from build123d import *

# Parameters (mm, degrees)
SKETCH1_W               = 100
SKETCH1_H               = 150
SKETCH1_W_2             = 88
SKETCH1_H_2             = 138
BOSS_EXTRUDE1_DEPTH     = 138.202315188
SKETCH2_R               = 40
CUT_EXTRUDE1_DEPTH      = 51
CUT_EXTRUDE1_DEPTH_BACK = 51


with BuildPart() as part:
    # Sketch1 → Boss-Extrude1 (new body)
    with BuildSketch(Plane.XY):
        Rectangle(SKETCH1_W, SKETCH1_H)
        Rectangle(SKETCH1_W_2, SKETCH1_H_2, mode=Mode.SUBTRACT)
    extrude(amount=BOSS_EXTRUDE1_DEPTH)

    # Sketch2 → Cut-Extrude1 (cut, two sides)
    with BuildSketch(Plane(origin=(0, 0, 0), x_dir=(0, 0, -1), z_dir=(1, 0, 0))) as cut_extrude1_sk:
        Circle(SKETCH2_R)
    extrude(amount=CUT_EXTRUDE1_DEPTH, mode=Mode.SUBTRACT)
    extrude(cut_extrude1_sk.sketch, amount=-CUT_EXTRUDE1_DEPTH_BACK, mode=Mode.SUBTRACT)


solid = part.part
Verification items for the finished model (mm, model axes). A direction names the side the tool comes from. Give positions to 0.01 mm unless a question says otherwise; leave off trailing zeros. Loops run counter-clockwise (first coordinate to the right, second up) from the corner with the lowest first, then second, coordinate; pieces in that order, holes last. Notation, with made-up numbers: (75.25, 50.25) - (104.25, 50.25) arc R31 cw to (104.25, 81.25) - close; hole circle Ø3 at (67.25, 45.25). An arc over 180 degrees is marked (long way). Write each question's results on one line, items separated by ' | '.
1) Sectioned sample at A-A on z = 24. Record the boundary of the cut face in (x, y), plus the area to 3 significant figures.
Solution:
outline: (-50, -75) - (50, -75) - (50, -32) - (44, -32) - (44, -69) - (-44, -69) - (-44, -32) - (-50, -32) - close; (-50, 32) - (-44, 32) - (-44, 69) - (44, 69) - (44, 32) - (50, 32) - (50, 75) - (-50, 75) - close | area: 2,090 mm2
2) Sectioned sample at B-B on y = -52. Record the boundary of the cut face in (x, z), plus the area to 3 significant figures.
Solution:
outline: (-50, 0) - (-44, 0) - (-44, 138.2) - (-50, 138.2) - close; (44, 0) - (50, 0) - (50, 138.2) - (44, 138.2) - close | area: 1,660 mm2
3) Sectioned sample at D-D on z = 66.5. Record the boundary of the cut face in (x, y).
Solution:
outline: (-50, -75) - (50, -75) - (50, 75) - (-50, 75) - close; hole (-44, -69) - (44, -69) - (44, 69) - (-44, 69) - close
4) Tool access check on faces 1 (the flat face through (-0.2, 69.2, 0)), 2 (the flat face through (44, -1, 83)). Record the directions out of +Z, -Z, +X, -X, +Y, -Y that give a thin tool (end or side, any length) a straight path to the whole face; none if there is none.
Solution:
face 1: -Z, +X, -X, +Y, -Y | face 2: +Z, -Z
5) Material ranges on L1, parallel to X at y = -1.5, z = 85.5; L2, parallel to Y at x = 32, z = 73.5; L3, parallel to Z at x = -45, y = 8.5, recorded low to high. Write a range as from..to.
Solution:
L1: -50..-44, 44..50 | L2: -75..-69, 69..75 | L3: 39.09..138.2
6) Mould release check, pull along X, two halves, no side actions. Record for faces 3 (the flat face through (-50, -1, 68)), 4 (the flat face through (50, -1, 68)), 5 (the flat face through (-44, -1, 83)), 6 (the flat face through (-1, -75, 68)): pulls with the +X half, pulls with the -X half, needs draft (parallel to the pull), parting line crosses it, or undercut.
Solution:
face 3: pulls with the -X half | face 4: pulls with the +X half | face 5: undercut | face 6: needs draft
7) Sectioned sample at C-C on x = -13.5. Record the boundary of the cut face in (y, z).
Solution:
outline: (-75, 0) - (-69, 0) - (-69, 138.2) - (-75, 138.2) - close; (69, 0) - (75, 0) - (75, 138.2) - (69, 138.2) - close
